Geometry: final body of the model. Coordinates: model frame, mm. A direction names the side the tool comes from. Give positions to 0.01 mm unless a question says otherwise; leave off trailing zeros. Write each loop counter-clockwise with the first axis right and the second up, starting at its lowest first coordinate (ties: lowest second). Pieces come first, ordered by that corner, then holes.
Autodesk Inventor part; units mm, degrees
ref_plane "YZ Plane" through (0, 0, 0) normal (1, 0, 0) x (0, 1, 0)
ref_plane "XZ Plane" through (0, 0, 0) normal (0, 1, 0) x (-1, 0, 0)
ref_plane "XY Plane" through (0, 0, 0) normal (0, 0, 1) x (1, 0, 0)
sketch "Sketch1" plane through (0, 0, 0) normal (0, 0, 1) x (1, 0, 0)
  line L0 (0, 0) -> (25.4, 0)
  line L1 (25.4, 0) -> (25.4, 25.4)
  line L2 (25.4, 25.4) -> (0, 25.4)
  line L3 (0, 25.4) -> (0, 0)
  line L4 (1.5875, 1.5875) -> (23.8125, 1.5875)
  line L5 (23.8125, 1.5875) -> (23.8125, 23.8125)
  line L6 (23.8125, 23.8125) -> (1.5875, 23.8125)
  line L7 (1.5875, 23.8125) -> (1.5875, 1.5875)
  dimension "d0" = 25.4
  dimension "d1" = 25.4
  dimension "d2" = 1.5875
extrude "Extrusion1" add sketch "Sketch1" along normal blind 165.1
sketch "Sketch2" plane through (0, 0, 0) normal (-1, 0, 0) x (0, 0, 1)
  arc A0 (33.3863, 14.478) -> (34.4023, 15.494) centre (33.3863, 15.494) ccw
  line L0 (34.4023, 15.494) -> (34.4023, 25.4)
  line L1 (34.4023, 25.4) -> (24.2423, 25.4)
  line L2 (24.2423, 25.4) -> (24.2423, 15.494)
  arc A1 (24.2423, 15.494) -> (25.2583, 14.478) centre (25.2583, 15.494) ccw
  line L3 (25.2583, 14.478) -> (33.3863, 14.478)
  circle A2 centre (29.3223, 19.05) radius 4.0005
extrude "Extrusion2" cut sketch "Sketch2" against normal blind 25.4 contours L3 A1 L2 L1 L0 A0 | A2
sketch "Sketch3" plane through (0, 0, 0) normal (0, -1, 0) x (1, 0, 0)
  circle A0 centre (12.7, 142.875) radius 3.3782
  circle A1 centre (12.7, 120.65) radius 3.3782
extrude "Extrusion3" cut sketch "Sketch3" against normal blind 25.4
sketch "Sketch4" plane through (0, 0, 0) normal (-1, 0, 0) x (0, 0, 1)
  circle A0 centre (152.4, 12.7) radius 3.3782
  circle A1 centre (101.6, 12.7) radius 3.3782
extrude "Extrusion4" cut sketch "Sketch4" against normal blind 25.4
properties part number "Camera Traffic Light Mount" material "Acetal Resin, White"
Item 1: Section B-B, the plane y = 12.7. Return the cut outline in (x, z), plus the area to 3 significant figures.
Found:
outline: (0, 0) - (1.59, 0) - (1.59, 98.22) - (0, 98.22) - close; (0, 104.98) - (1.59, 104.98) - (1.59, 149.02) - (0, 149.02) - close; (0, 155.78) - (1.59, 155.78) - (1.59, 165.1) - (0, 165.1) - close; (23.81, 0) - (25.4, 0) - (25.4, 98.22) - (23.81, 98.22) - close; (23.81, 104.98) - (25.4, 104.98) - (25.4, 149.02) - (23.81, 149.02) - close; (23.81, 155.78) - (25.4, 155.78) - (25.4, 165.1) - (23.81, 165.1) - close
area: 481 mm2
Item 2: Section C-C, the plane y = 21.25. Return the cut outline in (x, z), plus the area to 3 significant figures.
Found:
outline: (0, 0) - (1.59, 0) - (1.59, 24.24) - (0, 24.24) - close; (0, 34.4) - (1.59, 34.4) - (1.59, 165.1) - (0, 165.1) - close; (23.81, 0) - (25.4, 0) - (25.4, 24.24) - (23.81, 24.24) - close; (23.81, 34.4) - (25.4, 34.4) - (25.4, 165.1) - (23.81, 165.1) - close
area: 492 mm2
Item 3: Section A-A, the plane x = 12.7. Return the cut outline in (y, z), plus the area to 3 significant figures.
Found:
outline: (0, 0) - (1.59, 0) - (1.59, 117.27) - (0, 117.27) - close; (0, 124.03) - (1.59, 124.03) - (1.59, 139.5) - (0, 139.5) - close; (0, 146.25) - (1.59, 146.25) - (1.59, 165.1) - (0, 165.1) - close; (23.81, 0) - (25.4, 0) - (25.4, 24.24) - (23.81, 24.24) - close; (23.81, 34.4) - (25.4, 34.4) - (25.4, 117.27) - (23.81, 117.27) - close; (23.81, 124.03) - (25.4, 124.03) - (25.4, 139.5) - (23.81, 139.5) - close; (23.81, 146.25) - (25.4, 146.25) - (25.4, 165.1) - (23.81, 165.1) - close
area: 465 mm2
Item 4: Pull-direction query (Z, two-part tool) for faces 1 (the face through (24.595, 12.849, 98.225)), 2 (the face through (1, 13, 165.1)), 3 (the face through (13, 1.588, 81)); classes: +Z half, -Z half, draft (parallel to the pull), parting line (faces both ways), or undercut.
Found:
face 1: undercut
face 2: +Z half
face 3: draft
Item 5: Section D-D, the plane z = 120.65. Return the cut outline in (x, y), plus the area to 3 significant figures.
Found:
outline: (0, 0) - (9.32, 0) - (9.32, 1.59) - (1.59, 1.59) - (1.59, 23.81) - (9.32, 23.81) - (9.32, 25.4) - (0, 25.4) - close; (16.08, 0) - (25.4, 0) - (25.4, 25.4) - (16.08, 25.4) - (16.08, 23.81) - (23.81, 23.81) - (23.81, 1.59) - (16.08, 1.59) - close
area: 130 mm2
Item 6: Pin query (flat end, axial travel): pin 1 Ø3 at (x, z) = (20, 126.5) entering from -Y; pin 2 Ø0.8 at (x, z) = (24.5, 29) entering from +Y. Return the tip coordinate at first contact, or that it passes through.
Found:
pin 1: stops at y = 0
pin 2: stops at y = 14.48
Item 7: Reachability of faces 4 (the face through (13, 23.812, 12)), 5 (the face through (13, 24, 34.402)), 6 (the face through (14.3, 0.8, 139.9)) from +Z, -Z, +X, -X, +Y, -Y: full face, straight path, thin tool, end or side. Return the list, or none.
Found:
face 4: +Z, -Z
face 5: +X, -X, +Y
face 6: +Y, -Y
Item 8: Line query: L1, parallel to Z at x = 12.7, y = 24.5; L2, parallel to Z at x = 12.7, y = 0.7; L3, parallel to Y at x = 24.35, z = 152.4. Output: solid intervals per line, ascending.
Found:
L1: z = 0 to 24.24, 34.4 to 117.27, 124.03 to 139.5, 146.25 to 165.1
L2: z = 0 to 117.27, 124.03 to 139.5, 146.25 to 165.1
L3: y = 0 to 9.32, 16.08 to 25.4
